CAD build for the part. Positions are in the model's coordinates, mm. Face numbers are marked on the shaded views. A direction names the side the tool comes from. Coordinates: 2 decimals unless noted, no trailing zeros. Order: outer loops, then holes, each group sorted by start corner. A loop starts at its lowest first (then second) coordinate and runs counter-clockwise, first axis right, second up. Notation, with made-up numbers: (25.5, -9) - (58.5, -9) arc R8 cw to (58.5, 5) - close; hole circle Ø3 at (4, -22.75). An arc over 180 degrees is marked (long way). Write each question's results on one line, items separated by ' | '. Start each with the question number.
Q1. Band-saw the part on A-A, the plane z = 21. Write the cut outline in (x, y), then the cut area to 4 significant figures.
Q2. Band-saw the part on D-D, the plane z = -13. Write the cut outline in (x, y), then the cut area to 4 significant figures.
Q3. Band-saw the part on C-C, the plane x = 34.5. Write the cut outline in (y, z).
Q4. Pull direction X, two halves, no side cores. Call the marked faces 1, 2, 3 and 4: released by +X, released by -X, zero draft, split by the parting line, or undercut.
Q5. Wall check: probe 1 along Z at (x, y) = (-55, 22); probe 2 along X at (y, z) = (39.5, -27.5); probe 3 along X at (y, z) = (33, -40). Give the ranges that are in metal, low to high.
Q6. Pin check, flat tips, straight feed: P1, Ø3.5, axis at x = -43, z = 20.5, coming from the -Y side; P2, Ø2.5, axis at x = -42.5, z = -27.5, coming from the -Y side. Stop position of each tip, or through.
Q7. Which spindle directions (+Z, -Z, +X, -X, +Y, -Y) get a long thin tool onto all of the face, cutting with end or side? Do the marked faces 5 and 6. Say none if no direction does.
Q8. Band-saw the part on B-B, the plane y = 45.5. Count the separate pieces of the cut face and the enclosed holes in it, then the cut area to 3 significant figures.
```python
from build123d import *

# Parameters (mm, degrees)
SKETCH1_W             = 120
SKETCH1_H             = 90
BOSS_EXTRUDE1_DEPTH   = 50
M3_TAPPED_HOLE1_D     = 2.5
M3_TAPPED_HOLE1_DEPTH = 50
M3_TAPPED_HOLE1_TIP   = 0.751075774
SHELL2_T              = -2.5
FILLET2_R             = 2
CUT_EXTRUDE2_REACH    = 139.568
SKETCH13_R            = 5
CUT_EXTRUDE3_REACH    = 139.568
SKETCH14_R            = 1.75
SKETCH15_R            = 2
BOSS_EXTRUDE2_DEPTH   = 10
SKETCH16_R            = 1.5
CUT_EXTRUDE4_DEPTH    = 5


with BuildPart() as part:
    # Sketch1 → Boss-Extrude1 (new body)
    with BuildSketch(Plane(origin=(0, 0, 0), x_dir=(1, 0, 0), z_dir=(0, 1, 0))):
        Rectangle(SKETCH1_W, SKETCH1_H)
    extrude(amount=BOSS_EXTRUDE1_DEPTH)

    # M3 Tapped Hole1
    with Locations(Plane(origin=(0, 0, 0), x_dir=(-1, 0, 0), z_dir=(0, -1, 0))):
        with Locations((55, -40), (55, 40), (-55, 40), (-55, -40)):
            Hole(M3_TAPPED_HOLE1_D / 2, depth=M3_TAPPED_HOLE1_DEPTH)
            with Locations((0, 0, -(M3_TAPPED_HOLE1_DEPTH + M3_TAPPED_HOLE1_TIP / 2))):  # 118° drill point
                Cone(0, M3_TAPPED_HOLE1_D / 2, M3_TAPPED_HOLE1_TIP, mode=Mode.SUBTRACT)

    # Shell2
    shell2_openings = [part.faces().sort_by_distance(p)[0] for p in [
        (0, 0, 0),
    ]]
    offset(amount=SHELL2_T, openings=shell2_openings, kind=Kind.INTERSECTION)

    # Fillet2
    fillet2_edges = [part.edges().sort_by_distance(p)[0] for p in [
        (57.5, 23.75, -37.204915028),
        (-52.204915028, 23.75, -42.5),
        (-57.5, 23.75, 37.204915028),
        (52.204915028, 23.75, 42.5),
        (57.5, 23.75, 37.204915028),
        (52.204915028, 23.75, -42.5),
        (-57.5, 23.75, -37.204915028),
        (-52.204915028, 23.75, 42.5),
    ]]
    fillet(fillet2_edges, radius=FILLET2_R)

    # Sketch13 → Cut-Extrude2 (cut, up to next)
    with BuildSketch(Plane.ZY.offset(60), mode=Mode.PRIVATE) as cut_extrude2_sk1:
        with Locations((-19.268421651, 23.803658595)):
            Circle(SKETCH13_R)
    cut_extrude2_tool1 = extrude(cut_extrude2_sk1.sketch, amount=-CUT_EXTRUDE2_REACH, mode=Mode.PRIVATE) & part.part
    add(cut_extrude2_tool1.solids().sort_by_distance((-60, 23.803659, -19.268422))[0], mode=Mode.SUBTRACT)

    # Sketch14 → Cut-Extrude3 (cut, up to next)
    with BuildSketch(Plane(origin=(60, 0, 0), x_dir=(0, 0, -1), z_dir=(1, 0, 0)), mode=Mode.PRIVATE) as cut_extrude3_sk1:
        with Locations((-25.609467242, 29.516078094)):
            Circle(SKETCH14_R)
    cut_extrude3_tool1 = extrude(cut_extrude3_sk1.sketch, amount=-CUT_EXTRUDE3_REACH, mode=Mode.PRIVATE) & part.part
    add(cut_extrude3_tool1.solids().sort_by_distance((60, 29.516078, 25.609467))[0], mode=Mode.SUBTRACT)

    # Sketch15 → Boss-Extrude2 (add)
    with BuildSketch(Plane.XZ.offset(-47.5)):
        with Locations(Location((-42.5, -27.5, 0), (0, 0, 270))):
            Circle(SKETCH15_R)
        with Locations(Location((-42.5, 21, 0), (0, 0, 270))):
            Circle(SKETCH15_R)
        with Locations(Location((19.9, -27.5, 0), (0, 0, 270))):
            Circle(SKETCH15_R)
        with Locations(Location((19.9, 21, 0), (0, 0, 270))):
            Circle(SKETCH15_R)
    extrude(amount=BOSS_EXTRUDE2_DEPTH)

    # Sketch16 → Cut-Extrude4 (cut)
    with BuildSketch(Plane.XZ.offset(-37.5)):
        with Locations(Location((-42.5, 21, 0), (0, 0, 270))):
            Circle(SKETCH16_R)
        with Locations(Location((19.9, 21, 0), (0, 0, 270))):
            Circle(SKETCH16_R)
        with Locations(Location((-42.5, -27.5, 0), (0, 0, 270))):
            Circle(SKETCH16_R)
        with Locations(Location((19.9, -27.5, 0), (0, 0, 270))):
            Circle(SKETCH16_R)
    extrude(amount=-CUT_EXTRUDE4_DEPTH, mode=Mode.SUBTRACT)


solid = part.part
```
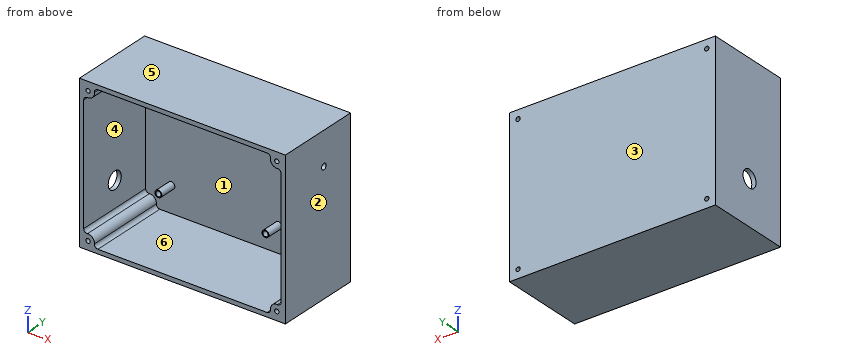
Results below:
1) outline: (-60, 0) - (-57.5, 0) - (-57.5, 47.5) - (-44.5, 47.5) - (-44.5, 37.5) - (-44, 37.5) - (-44, 42.5) - (-41, 42.5) - (-41, 37.5) - (-40.5, 37.5) - (-40.5, 47.5) - (17.9, 47.5) - (17.9, 37.5) - (18.4, 37.5) - (18.4, 42.5) - (21.4, 42.5) - (21.4, 37.5) - (21.9, 37.5) - (21.9, 47.5) - (57.5, 47.5) - (57.5, 0) - (60, 0) - (60, 50) - (-60, 50) - close | area: 587.5 mm²
2) outline: (-60, 0) - (-57.5, 0) - (-57.5, 47.5) - (57.5, 47.5) - (57.5, 0) - (60, 0) - (60, 50) - (-60, 50) - close | area: 537.5 mm²
3) outline: (0, -45) - (50, -45) - (50, 45) - (0, 45) - (0, 42.5) - (47.5, 42.5) - (47.5, -42.5) - (0, -42.5) - close
4) face 1: undercut | face 2: released by +X | face 3: zero draft | face 4: undercut
5) probe 1: z = -45 to -41.25, -38.75 to -36.25, 36.25 to 38.75, 41.25 to 45 | probe 2: x = -60 to -57.5, -44.5 to -44, -41 to -40.5, 17.9 to 18.4, 21.4 to 21.9, 57.5 to 60 | probe 3: x = -60 to -56.25, -53.75 to -51.25, 51.25 to 53.75, 56.25 to 60
6) P1: stops at y = 37.5 | P2: stops at y = 42.5
7) face 5: +Z, +X, -X, +Y, -Y | face 6: -Y
8) separate pieces: 5 | enclosed holes: 5 | area: 1,210 mm²
